```python
from build123d import *

# Parameters (mm, degrees)
SKETCH1_R           = 5
BOSS_EXTRUDE1_DEPTH = 5
SKETCH2_R           = 2.4
BOSS_EXTRUDE2_DEPTH = 27.5
CHAMFER1_SIZE       = 2.5
SKETCH3_R           = 1.25
CUT_EXTRUDE1_DEPTH  = 34.260336739


with BuildPart() as part:
    # Sketch1 → Boss-Extrude1 (new body)
    with BuildSketch(Plane.XY):
        Circle(SKETCH1_R)
    extrude(amount=BOSS_EXTRUDE1_DEPTH)

    # Sketch2 → Boss-Extrude2 (add)
    with BuildSketch(Plane.XY.offset(5)):
        Circle(SKETCH2_R)
    extrude(amount=BOSS_EXTRUDE2_DEPTH)

    # Chamfer1
    chamfer1_edges = [part.edges().sort_by_distance(p)[0] for p in [
        (-5, 0, 0),
    ]]
    chamfer(chamfer1_edges, length=CHAMFER1_SIZE)

    # Sketch3 → Cut-Extrude1 (cut, through all)
    with BuildSketch(Plane.XY.offset(32.5)):
        Circle(SKETCH3_R)
    extrude(amount=-CUT_EXTRUDE1_DEPTH, mode=Mode.SUBTRACT)


solid = part.part
```
Build history of the part. All positions in model axes, mm. A direction names the side the tool comes from. Round coordinates to 2 decimals unless told otherwise and drop trailing zeros. Order: outer loops, then holes, each group sorted by start corner. A loop starts at its lowest first (then second) coordinate and runs counter-clockwise, first axis right, second up. Notation, with made-up numbers: (50.5, 58.25) -> (85.5, 58.25) arc R20 ccw to (85.5, 97.25) -> close; hole circle Ø4 at (-35, 29). An arc over 180 degrees is marked (long way). Answer in a Markdown table with one row per item.
1) Band-saw the part on C-C on z = 9.5. Give the cut face in (x, y), and give its area (3 significant figures).
Values:
| item | result |
|---|---|
| outline | circle Ø4.8 at (0, 0); hole circle Ø2.5 at (0, 0) |
| area | 13.2 mm2 |
2) Pin check, flat tips, straight feed: P1, Ø1, axis at x = 2, z = 28.5, coming from the -Y side; P2, Ø6, axis at x = -3.5, z = 27.5, coming from the +Y side. Stop position of each tip, or through.
Values:
| item | result |
|---|---|
| P1 | y = -1.87 |
| P2 | y = 2.35 |
3) Which spindle directions (+Z, -Z, +X, -X, +Y, -Y) get a long thin tool onto all of the face, cutting with end or side? Do faces 1 (the flat face through (-1.2, 2.3, 5)), 2 (the flat face through (1, -1, 32.5)). Say none if no direction does.
Values:
| item | result |
|---|---|
| face 1 | +Z |
| face 2 | +Z, +X, -X, +Y, -Y |
4) Band-saw the part on A-A on y = 0. Give the cut face in (x, z).
Values:
| item | result |
|---|---|
| outline | (-5, 2.5) -> (-2.5, 0) -> (-1.25, 0) -> (-1.25, 32.5) -> (-2.4, 32.5) -> (-2.4, 5) -> (-5, 5) -> close; (1.25, 0) -> (2.5, 0) -> (5, 2.5) -> (5, 5) -> (2.4, 5) -> (2.4, 32.5) -> (1.25, 32.5) -> close |
5) Wall check: L1, parallel to Y at x = 0, z = 12; L2, parallel to Y at x = 0.5, z = 23.5; L3, parallel to X at y = 1, z = 5.5. Give the ranges that are in metal, low to high.
Values:
| item | result |
|---|---|
| L1 | -2.4 to -1.25, 1.25 to 2.4 |
| L2 | -2.35 to -1.15, 1.15 to 2.35 |
| L3 | -2.18 to -0.75, 0.75 to 2.18 |
